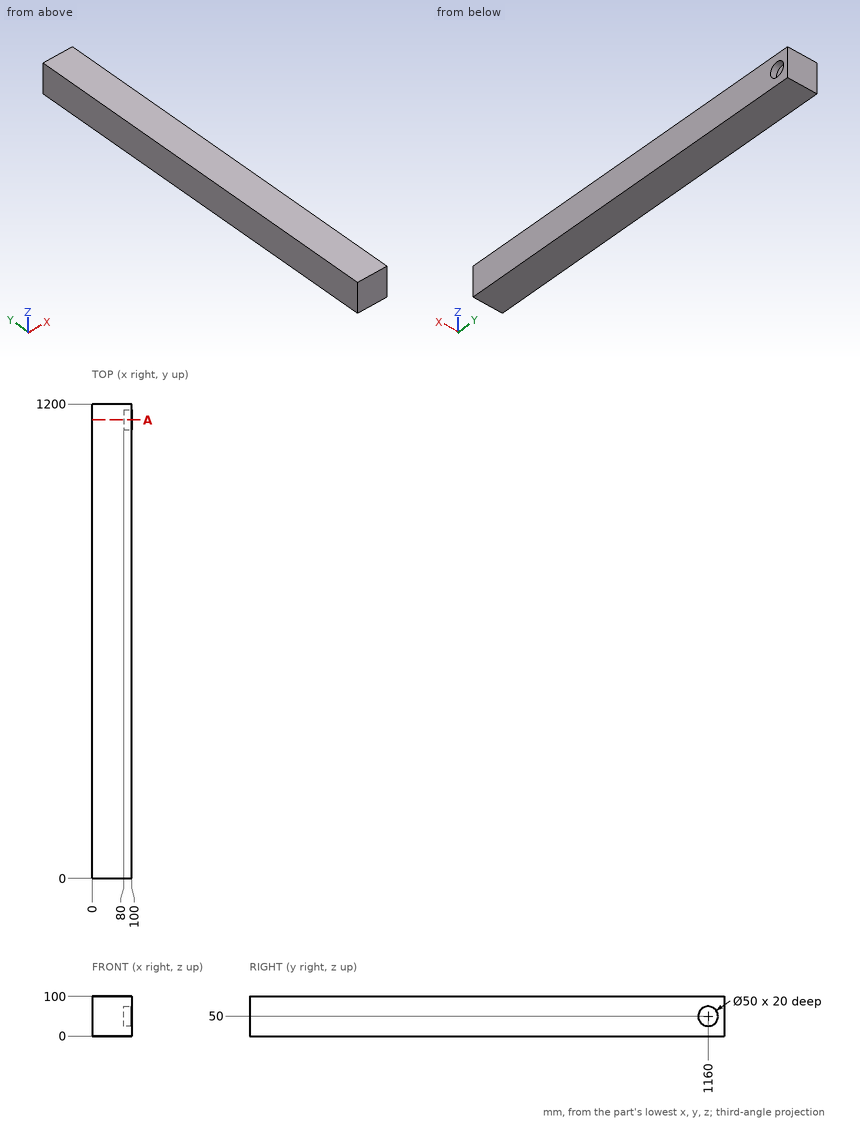
The figure shows three views and two pictorial views of one solid part (mm, origin at its lowest corner). Answer the questions. Coordinates: 2 decimals unless noted, no trailing zeros. Loops run counter-clockwise (first coordinate to the right, second up) from the corner with the lowest first, then second, coordinate; pieces in that order, holes last.
(1) The part is cut by section A-A (y = 1160). Determine the outline of the cut face in (x, z).
Solution:
outline: (0, 0) - (100, 0) - (100, 25) - (80, 25) - (80, 75) - (100, 75) - (100, 100) - (0, 100) - close
(2) Consider line 1 along Z through (x, y) = (95.5, 1160); line 2 along Y through (x, z) = (89, 50); line 3 along Y through (x, z) = (84.5, 70.5). Determine where each line is inside the solid, lowest interval first.
Solution:
line 1: z = 0 to 25, 75 to 100
line 2: y = 0 to 1135, 1185 to 1200
line 3: y = 0 to 1145.69, 1174.31 to 1200
(3) A flat-ended cylindrical pin translates along its axis: pin 1 Ø2 at (x, y) = (51.5, 1034.5) entering from -Z. Find the tip coordinate at first contact, or state that the pin passes through.
Solution:
pin 1: stops at z = 0
